from build123d import *

# Parameters (mm, degrees)
SKETCH1_W           = 82
SKETCH1_H           = 52
BOSS_EXTRUDE1_DEPTH = 2
FILLET1_R           = 2
CUT_EXTRUDE1_DEPTH  = 49.590122453
SKETCH3_R           = 2
CUT_EXTRUDE2_DEPTH  = 49.590122453


with BuildPart() as part:
    # Sketch1 → Boss-Extrude1 (new body)
    with BuildSketch(Plane.XY):
        Rectangle(SKETCH1_W, SKETCH1_H)
    extrude(amount=BOSS_EXTRUDE1_DEPTH)

    # Fillet1
    fillet1_edges = [part.edges().sort_by_distance(p)[0] for p in [
        (-41, 26, 1),
        (41, 26, 1),
        (41, -26, 1),
        (-41, -26, 1),
    ]]
    fillet(fillet1_edges, radius=FILLET1_R)

    # Sketch2 → Cut-Extrude1 (cut, through all)
    with BuildSketch(Plane.XY.offset(2)):
        with BuildLine():
            Line((-18.5, 20.5), (12.5, 20.5))
            ThreePointArc((12.5, 20.5), (14, 19), (12.5, 17.5))
            Line((12.5, 17.5), (-18.5, 17.5))
            ThreePointArc((-18.5, 17.5), (-20, 19), (-18.5, 20.5))
        make_face()
        with BuildLine():
            Line((-18.5, 15), (12.5, 15))
            ThreePointArc((12.5, 15), (14, 13.5), (12.5, 12))
            Line((12.5, 12), (-18.5, 12))
            ThreePointArc((-18.5, 12), (-20, 13.5), (-18.5, 15))
        make_face()
        with BuildLine():
            Line((-18.5, 9.5), (12.5, 9.5))
            ThreePointArc((12.5, 9.5), (14, 8), (12.5, 6.5))
            Line((12.5, 6.5), (-18.5, 6.5))
            ThreePointArc((-18.5, 6.5), (-20, 8), (-18.5, 9.5))
        make_face()
        with BuildLine():
            Line((-18.5, 4), (12.5, 4))
            ThreePointArc((12.5, 4), (14, 2.5), (12.5, 1))
            Line((12.5, 1), (-18.5, 1))
            ThreePointArc((-18.5, 1), (-20, 2.5), (-18.5, 4))
        make_face()
    extrude(amount=-CUT_EXTRUDE1_DEPTH, mode=Mode.SUBTRACT)

    # Sketch3 → Cut-Extrude2 (cut, through all)
    with BuildSketch(Plane.XY.offset(2)):
        with Locations((37.5, 22.5)):
            Circle(SKETCH3_R)
        with Locations((-37.5, 22.5)):
            Circle(SKETCH3_R)
        with Locations((37.5, -22.5)):
            Circle(SKETCH3_R)
        with Locations((-37.5, -22.5)):
            Circle(SKETCH3_R)
    extrude(amount=-CUT_EXTRUDE2_DEPTH, mode=Mode.SUBTRACT)


solid = part.part
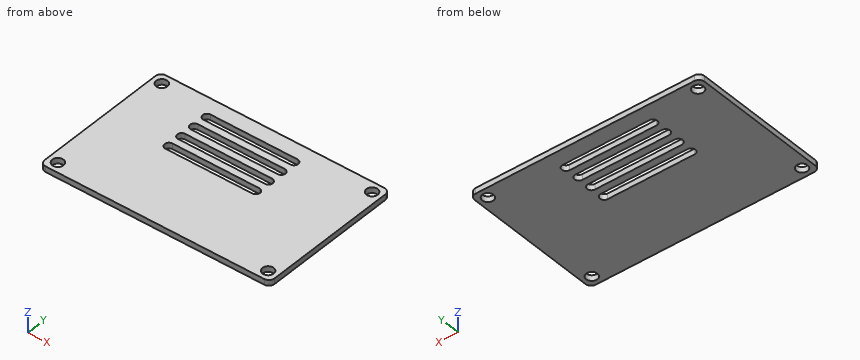
Geometry check sheet. Reference: the model listing, model coordinates, mm. Give positions to 0.01 mm unless a question says otherwise; leave off trailing zeros. Loops run counter-clockwise (first coordinate to the right, second up) from the corner with the lowest first, then second, coordinate; pieces in that order, holes last. Notation, with made-up numbers: (52, 26) -> (66, 26) arc R25 cw to (66, 51) -> close; hole circle Ø9 at (58.25, 43.5). An arc over 180 degrees is marked (long way). Answer in a Markdown table with one row per item. Add a question column.
1) Cross-section at D-D on z = 0.8. State how many separate pieces and enclosed holes the cut face has, and give its area (3 significant figures).
2) Cross-section at C-C on y = 22.5. Record the boundary of the cut face in (x, z).
3) Cross-section at B-B on x = -37.5. Record the boundary of the cut face in (y, z).
4) Cross-section at A-A on y = 2.5. Record the boundary of the cut face in (x, z).
5) Material ranges on probe 1 along Y at (x, z) = (-37.5, 0.85); probe 2 along Y at (x, z) = (-9.5, 1.4); probe 3 along Y at (x, z) = (-19, 1), recorded low to high. Write a range as from..to.
Outcome:
| question | item | result |
|---|---|---|
| 1 | separate pieces | 1 |
| 1 | enclosed holes | 8 |
| 1 | area | 3,810 mm^2 |
| 2 | outline | (-41, 0) -> (-39.5, 0) -> (-39.5, 2) -> (-41, 2) -> close; (-35.5, 0) -> (35.5, 0) -> (35.5, 2) -> (-35.5, 2) -> close; (39.5, 0) -> (41, 0) -> (41, 2) -> (39.5, 2) -> close |
| 3 | outline | (-26, 0) -> (-24.5, 0) -> (-24.5, 2) -> (-26, 2) -> close; (-20.5, 0) -> (20.5, 0) -> (20.5, 2) -> (-20.5, 2) -> close; (24.5, 0) -> (26, 0) -> (26, 2) -> (24.5, 2) -> close |
| 4 | outline | (-41, 0) -> (-20, 0) -> (-20, 2) -> (-41, 2) -> close; (14, 0) -> (41, 0) -> (41, 2) -> (14, 2) -> close |
| 5 | probe 1 | y = -26..-24.5, -20.5..20.5, 24.5..26 |
| 5 | probe 2 | y = -26..1, 4..6.5, 9.5..12, 15..17.5, 20.5..26 |
| 5 | probe 3 | y = -26..1.09, 3.91..6.59, 9.41..12.09, 14.91..17.59, 20.41..26 |
